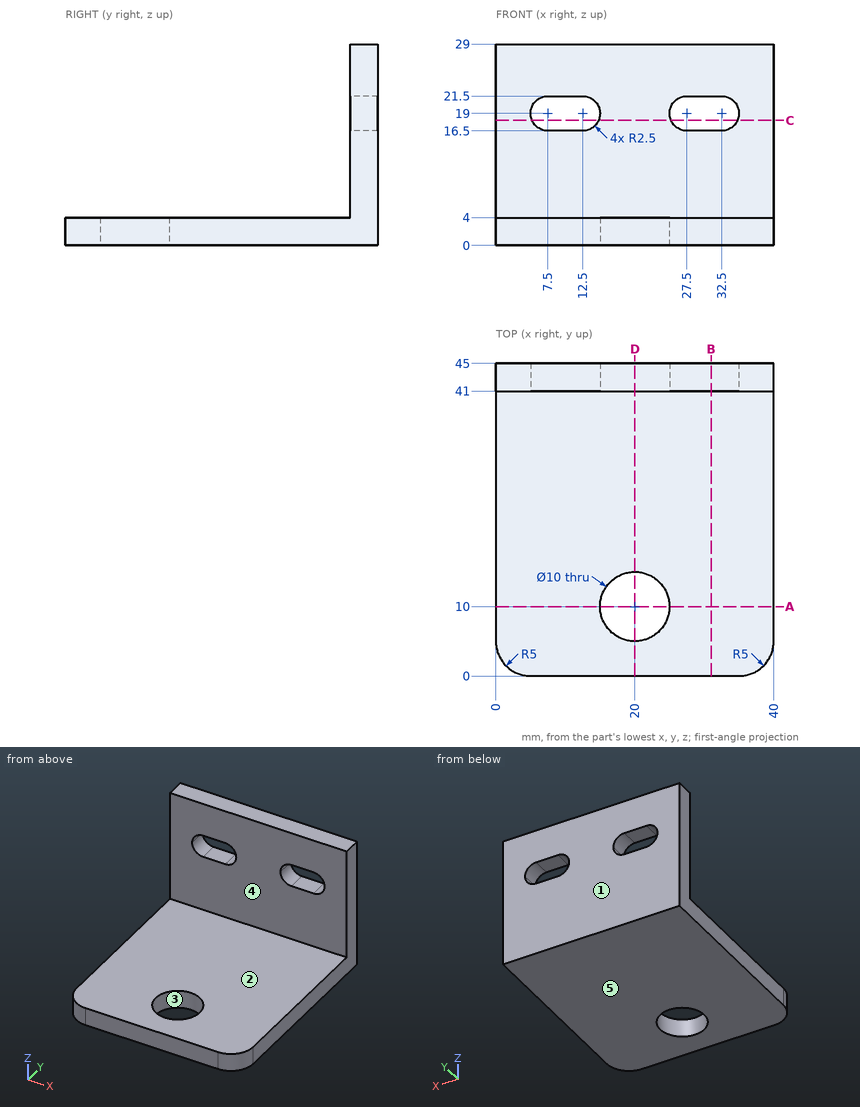
Job drawing, mm, ordinate dimensions from the low corner. One solid piece. A direction names the side the tool comes from. Give positions to 0.01 mm unless a question says otherwise; leave off trailing zeros. Write each loop counter-clockwise with the first axis right and the second up, starting at its lowest first coordinate (ties: lowest second). Pieces come first, ordered by that corner, then holes. Notation, with made-up numbers: M 64.5,65.25 L 107.5,65.25 A22 ccw 107.5,78.25 Z; hole C 10,-38.5 d6. An arc over 180 degrees is marked long. Put each result on its own line as item: value. Start each with the question number.
(1) Band-saw the part on A-A, the plane y = 10. Write the cut outline in (x, z), and give its area (3 significant figures).
(2) Band-saw the part on C-C, the plane z = 18. Write the cut outline in (x, y), and give its area (3 significant figures).
(3) Band-saw the part on B-B, the plane x = 31. Write the cut outline in (y, z), and give its area (3 significant figures).
(4) Probe L1, parallel to Y at x = 20, z = 2.8; L2, parallel to Z at x = 8, y = 17; L3, parallel to Y at x = 34, z = 27.5. List the from-to ranges inside material, lowest first.
(5) Mould opens along Y. For the marked faces 3, 4 and 5 say: +Y half, -Y half, draft (parallel to the pull), parting line (faces both ways), or undercut.
(6) Which spindle directions (+Z, -Z, +X, -X, +Y, -Y) get a long thin tool onto all of the face, cutting with end or side? Do the marked faces 1 and 2. Say none if no direction does.
(7) Band-saw the part on D-D, the plane x = 20. Write the cut outline in (y, z), and give its area (3 significant figures).
(8) Flat gauge pins, fed straight in: pin 1 Ø1 at (x, y) = (30.5, 35.5) entering from +Z; pin 2 Ø8 at (x, z) = (32.5, 14) entering from -Y; pin 3 Ø9 at (x, y) = (20, 10) entering from -Z. Where does each tip first touch, or does it go through?
Response values:
1. outline: M 0,0 L 15,0 L 15,4 L 0,4 Z; M 25,0 L 40,0 L 40,4 L 25,4 Z
1. area: 120 mm2
2. outline: M 0,41 L 5.21,41 L 5.21,45 L 0,45 Z; M 14.79,41 L 25.21,41 L 25.21,45 L 14.79,45 Z; M 34.79,41 L 40,41 L 40,45 L 34.79,45 Z
2. area: 83.3 mm2
3. outline: M 0,0 L 45,0 L 45,16.5 L 41,16.5 L 41,4 L 0,4 Z; M 41,21.5 L 45,21.5 L 45,29 L 41,29 Z
3. area: 260 mm2
4. L1: y = 0 to 5, 15 to 45
4. L2: z = 0 to 4
4. L3: y = 41 to 45
5. face 3: undercut
5. face 4: -Y half
5. face 5: draft
6. face 1: +Z, -Z, +X, -X, +Y
6. face 2: +Z, +X, -X, -Y
7. outline: M 0,0 L 5,0 L 5,4 L 0,4 Z; M 15,0 L 45,0 L 45,29 L 41,29 L 41,4 L 15,4 Z
7. area: 240 mm2
8. pin 1: stops at z = 4
8. pin 2: stops at y = 41
8. pin 3: passes through
